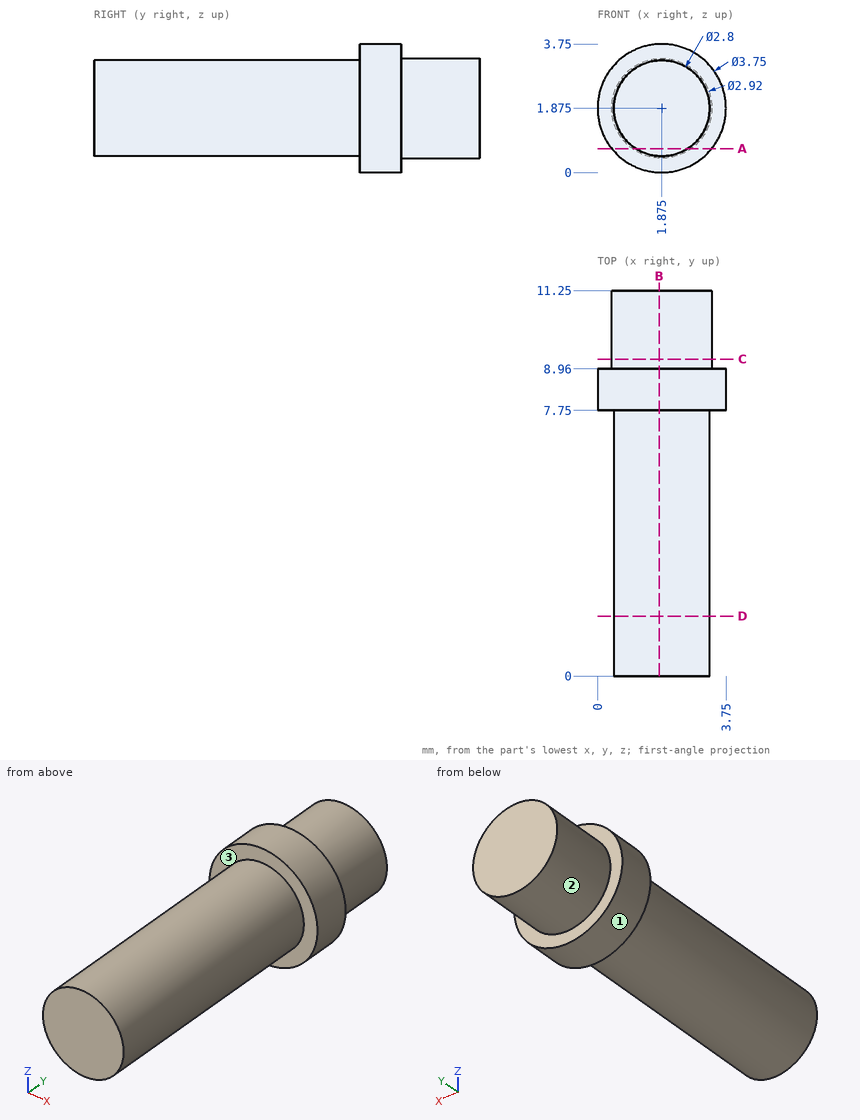
Part print with two shaded views. Sizes in mm from the minimum x, y, z corner. A direction names the side the tool comes from. Coordinates: 2 decimals unless noted, no trailing zeros. Loops run counter-clockwise (first coordinate to the right, second up) from the corner with the lowest first, then second, coordinate; pieces in that order, holes last. Notation, with made-up numbers: (-17, 7.5) -> (42, 7.5) arc R15 ccw to (42, 21.5) -> close; hole circle Ø4 at (-30.5, 3.5). An arc over 180 degrees is marked (long way). Answer as a JSON object with one key per item and string values.
Q1. 3-axis set-ups, long thin cutter, end or side, ignore diameter. For the marked faces 1, 2 and 3: which of +Z, -Z, +X, -X, +Y, -Y reach the whole face in a straight line?
Report:
{"face 1": "+Y, -Y", "face 2": "+Y", "face 3": "-Y"}
Q2. Flat gauge pins, fed straight in: P1, Ø1, axis at x = 0.5, z = 0.5, coming from the -Y side; P2, Ø1, axis at x = 1, y = 3.5, coming from the +Z side. Where does each tip first touch, or does it go through?
Report:
{"P1": "stops at y = 7.75", "P2": "stops at z = 3.22"}
Q3. Cut at D-D (y = 1.75). List the corners of the cut face in (x, z) (3 decimals).
Report:
{"outline": "circle Ø2.8 at (1.875, 1.875)"}
Q4. Cut at B-B (x = 1.8). List the corners of the cut face in (y, z), and give its area (3 significant figures).
Report:
{"outline": "(0, 0.48) -> (7.75, 0.48) -> (7.75, 0) -> (8.96, 0) -> (8.96, 0.42) -> (11.25, 0.42) -> (11.25, 3.33) -> (8.96, 3.33) -> (8.96, 3.75) -> (7.75, 3.75) -> (7.75, 3.27) -> (0, 3.27) -> close", "area": "32.9 mm2"}
Q5. Cut at A-A (z = 0.7). List the corners of the cut face in (x, y), and give its area (3 significant figures).
Report:
{"outline": "(0.41, 7.75) -> (1.11, 7.75) -> (1.11, 0) -> (2.64, 0) -> (2.64, 7.75) -> (3.34, 7.75) -> (3.34, 8.96) -> (2.74, 8.96) -> (2.74, 11.25) -> (1.01, 11.25) -> (1.01, 8.96) -> (0.41, 8.96) -> close", "area": "19.3 mm2"}
Q6. Probe probe 1 along Y at (x, z) = (0.8, 0.55); probe 2 along Z at (x, y) = (1.95, 6); probe 3 along Z at (x, y) = (1.3, 6.5). List the from-to ranges inside material, lowest first.
Report:
{"probe 1": "y = 7.75 to 8.96", "probe 2": "z = 0.48 to 3.27", "probe 3": "z = 0.6 to 3.15"}
Q7. Cut at C-C (y = 9.25). List the corners of the cut face in (x, z) (3 decimals), and give its area (3 significant figures).
Report:
{"outline": "circle Ø2.92 at (1.875, 1.875)", "area": "6.70 mm2"}
